from build123d import *

# Parameters (mm, degrees)
SKETCH5_R           = 3.175
BOSS_EXTRUDE3_DEPTH = 69.85
CHAMFER1_SIZE       = 0.9525
BOSS_EXTRUDE4_DEPTH = 3.96875
SKETCH8_OUTSIDE_W   = 287.44
SKETCH8_OUTSIDE_H   = 289.16
SKETCH8_OUTSIDE_R   = 5.55625
CUT_EXTRUDE3_DEPTH  = 74.81875
CUT_EXTRUDE3_TAPER  = 60
CUT_EXTRUDE4_DEPTH  = 0.254
CIRPATTERN1_COUNT   = 3


with BuildPart() as part:
    # Sketch5 → Boss-Extrude3 (new body)
    with BuildSketch(Plane(origin=(36.909375, 0, 0), x_dir=(0, 0, -1), z_dir=(1, 0, 0))):
        Circle(SKETCH5_R)
    extrude(amount=-BOSS_EXTRUDE3_DEPTH)

    # Chamfer1
    chamfer1_edges = [part.edges().sort_by_distance(p)[0] for p in [
        (36.909375, 0, 3.175),
    ]]
    chamfer(chamfer1_edges, length=CHAMFER1_SIZE)

    # Sketch11 → Revolve1 (revolve)
    with BuildSketch(Plane.XY):
        Polygon((-32.940625, 3.175), (-32.940625, 0), (21.034375, 0), (17.859375, 3.175), align=None)
    revolve(axis=Axis((-32.940625, 0, 0), (1, 0, 0)))

    # Sketch6 → Boss-Extrude4 (add)
    with BuildSketch(Plane.ZY.offset(32.940625)):
        Polygon((5.55625, 3.207902433), (0, 6.415804866), (-5.55625, 3.207902433), (-5.55625, -3.207902433), (0, -6.415804866), (5.55625, -3.207902433), align=None)
    extrude(amount=BOSS_EXTRUDE4_DEPTH)

    # Sketch8 outside → Cut-Extrude3 (cut, through all)
    with BuildSketch(Plane.ZY.offset(36.909375)):
        Rectangle(SKETCH8_OUTSIDE_W, SKETCH8_OUTSIDE_H)
        Circle(SKETCH8_OUTSIDE_R, mode=Mode.SUBTRACT)
    extrude(amount=-CUT_EXTRUDE3_DEPTH, taper=CUT_EXTRUDE3_TAPER, mode=Mode.SUBTRACT)

    # Sketch12 → Cut-Extrude4 (cut)
    with BuildSketch(Plane.ZY.offset(36.909375)):
        with BuildLine():
            Line((0.1666875, 4.2783125), (0.1666875, 2.3891875))
            ThreePointArc((0.1666875, 2.3891875), (0, 2.2225), (-0.1666875, 2.3891875))
            Line((-0.1666875, 2.3891875), (-0.1666875, 4.2783125))
            ThreePointArc((-0.1666875, 4.2783125), (0, 4.445), (0.1666875, 4.2783125))
        make_face()
    cut_extrude4 = extrude(amount=-CUT_EXTRUDE4_DEPTH, mode=Mode.SUBTRACT)

    # CirPattern1: Cut-Extrude4 ×3 about axis
    cirpattern1_axis = Axis((0, 0, 0), (1, 0, 0))
    for i in range(1, CIRPATTERN1_COUNT):
        add(cut_extrude4.rotate(cirpattern1_axis, i * 360 / CIRPATTERN1_COUNT), mode=Mode.SUBTRACT)


solid = part.part
Work out the finished part from the listing and answer in its coordinate system (mm). A direction names the side the tool comes from. Coordinates: 2 decimals unless noted, no trailing zeros. Order: outer loops, then holes, each group sorted by start corner. A loop starts at its lowest first (then second) coordinate and runs counter-clockwise, first axis right, second up. Notation, with made-up numbers: (21.5, 46) - (73.5, 46) arc R22 cw to (73.5, 80) - close; hole circle Ø4 at (32.5, 37.5). An arc over 180 degrees is marked (long way). Put each result on its own line as item: value. Start each with the question number.
1) Find section A-A (x = -17). Give the vertices of the cut face in (y, z) (3 decimals).
2) Flat-ended cylindrical pins translate along their axes: pin 1 (6 mm diameter, centred on x = -4.5, z = 1.5, fed in from +Y) (3 decimals); pin 2 (2 mm diameter, centred on x = -1, z = 1, fed in from -Y) (3 decimals); pin 3 (3 mm diameter, centred on x = -6.5, y = -4, fed in from +Z); pin 4 (3 mm diameter, centred on y = 0, z = 2.5, fed in from +X). Find the tip coordinate at first contact, or state that the pin passes through.
3) For faces 5 (the flat face through (-32.941, -3, -3)), 6 (the flat face through (-34.897, -4.834, 2.739)), determine the directions among +Z, -Z, +X, -X, +Y, -Y from which every point of the face is accessible in a straight line to the end or side of a thin tool.
4) Find the intervals of material crossed by line 1 (Y direction, x = 8, z = 0.25); line 2 (X direction, y = 2.75, z = -2.5); line 3 (Y direction, x = 11, z = -0.75), in increasing order. Write a range as from..to.
5) For a pull along Y with two mould halves and no side action, classify faces 1 (the flat face through (-36.655, -1.67, -2.9)), 2 (the flat face through (-36.655, -1.68, 2.9)), 3 (the conical face through (-36.789, 5.765, -0.014)), 4 (the conical face through (-36.79, -2.89, -4.99)) as released by +Y, released by -Y, zero draft, split by the parting line, or undercut.
Results list:
1. outline: circle Ø6.35 at (0, 0)
2. pin 1: stops at y = 3.175
2. pin 2: stops at y = -3.175
2. pin 3: stops at z = 1.96
2. pin 4: stops at x = 36.91
3. face 5: +X
3. face 6: +Z, +X, -X, -Y
4. line 1: y = -3.17..3.17
4. line 2: x = -36.91..-32.94
4. line 3: y = -3.09..3.09
5. face 1: undercut
5. face 2: undercut
5. face 3: released by +Y
5. face 4: released by -Y
